Build history of the part. All positions in model axes, mm. Give positions to 0.01 mm unless a question says otherwise; leave off trailing zeros. Order: outer loops, then holes, each group sorted by start corner. A loop starts at its lowest first (then second) coordinate and runs counter-clockwise, first axis right, second up. Notation, with made-up numbers: (65, 0.25) - (88, 0.25) arc R36 cw to (88, 34.25) - close; hole circle Ø8 at (18.5, 70). An arc over 180 degrees is marked (long way). Write each question's results on one line, items separated by ' | '. Start each with the question number.
1) Cut at B-B on z = -7. List the corners of the cut face in (x, y).
2) Cut at C-C on y = 0. State how many separate pieces and enclosed holes the cut face has, plus the area to 3 significant figures.
3) Drill centre lines: line 1 along Z through (x, y) = (54, 10.75); line 2 along Z through (x, y) = (25.4, 11.6). Where is each one in solid material? Low to high. Write a range as from..to.
4) Two-plate mould, pull along Z, no slides. Class faces 1 (the face through (2, -12.7, -3)), 2 (the face through (-48.5, 11.9, 0.95)): +Z half, -Z half, draft (parallel to the pull), parting line (faces both ways), or undercut.
5) Drop a flat-ended pin along its axis: pin 1 Ø5.5 at (x, y) = (101.6, 0) entering from -Z. Give the stop position or say it passes through.
6) Cut at A-A on x = -101.6. List the corners of the cut face in (y, z).
from build123d import *

# Parameters (mm, degrees)
SKETCH1_W             = 25.4
SKETCH1_H             = 25.4
SKETCH1_W_2           = 22.225
SKETCH1_H_2           = 22.225
BOSS_EXTRUDE1_DEPTH   = 139.7
SKETCH3_W             = 2.4892
SKETCH3_H             = 25.4
SKETCH3_AT_POINT_2_W  = 2.4892
SKETCH3_AT_POINT_2_H  = 25.4
LPATTERN1_START       = -12.7
LPATTERN1_OUTLINE_R   = 2.4892
LPATTERN1_DEPTH       = 25.4
LPATTERN1_2_OUTLINE_R = 2.4892
LPATTERN1_2_DEPTH     = 25.4


# Read off the part's stored shape, not the designer's step: LPattern1
with BuildPart() as part:
    # Sketch1 → Boss-Extrude1 (new, symmetric)
    with BuildSketch(Plane(origin=(0, 0, 0), x_dir=(0, 0, -1), z_dir=(1, 0, 0))):
        Rectangle(SKETCH1_W, SKETCH1_H)
        Rectangle(SKETCH1_W_2, SKETCH1_H_2, mode=Mode.SUBTRACT)
    extrude(amount=BOSS_EXTRUDE1_DEPTH, both=True)

    # Sketch3 → #9 (0.196) Diameter Hole1 (revolve, cut)
    with BuildSketch(Plane(origin=(127, 12.7, 0), x_dir=(0, 0, 1), z_dir=(1, 0, 0))):
        with Locations((1.2446, 12.7)):
            Rectangle(SKETCH3_W, SKETCH3_H)
    revolve(axis=Axis((127, 19.05, 0), (0, -1, 0)), mode=Mode.SUBTRACT)

    # Sketch3 at point 2 (carried to point 2, square into its face) → #9 (0.196) Diameter Hole1 at 2 (revolve, cut)
    with BuildSketch(Plane(origin=(127, 0, 12.7), x_dir=(0, -1, 0), z_dir=(1, 0, 0))):
        with Locations((1.2446, 12.7)):
            Rectangle(SKETCH3_AT_POINT_2_W, SKETCH3_AT_POINT_2_H)
    revolve(axis=Axis((127, 0, 19.05), (0, 0, -1)), mode=Mode.SUBTRACT)

    # LPattern1 outline → LPattern1 (cut)
    with BuildSketch(Plane.XY.offset(LPATTERN1_START)):
        with Locations((101.6, 0)):
            Circle(LPATTERN1_OUTLINE_R)
        with Locations((76.2, 0)):
            Circle(LPATTERN1_OUTLINE_R)
        with Locations((50.8, 0)):
            Circle(LPATTERN1_OUTLINE_R)
        with Locations((25.4, 0)):
            Circle(LPATTERN1_OUTLINE_R)
        Circle(LPATTERN1_OUTLINE_R)
        with Locations((-25.4, 0)):
            Circle(LPATTERN1_OUTLINE_R)
        with Locations((-50.8, 0)):
            Circle(LPATTERN1_OUTLINE_R)
        with Locations((-76.2, 0)):
            Circle(LPATTERN1_OUTLINE_R)
        with Locations((-101.6, 0)):
            Circle(LPATTERN1_OUTLINE_R)
        with Locations((-127, 0)):
            Circle(LPATTERN1_OUTLINE_R)
    extrude(amount=LPATTERN1_DEPTH, mode=Mode.SUBTRACT)

    # LPattern1 2 outline → LPattern1 2 (cut)
    with BuildSketch(Plane(origin=(0, 0, 0), x_dir=(1, 0, 0), z_dir=(0, 1, 0)).offset(LPATTERN1_START)):
        with Locations((101.6, 0)):
            Circle(LPATTERN1_2_OUTLINE_R)
        with Locations((76.2, 0)):
            Circle(LPATTERN1_2_OUTLINE_R)
        with Locations((50.8, 0)):
            Circle(LPATTERN1_2_OUTLINE_R)
        with Locations((25.4, 0)):
            Circle(LPATTERN1_2_OUTLINE_R)
        Circle(LPATTERN1_2_OUTLINE_R)
        with Locations((-25.4, 0)):
            Circle(LPATTERN1_2_OUTLINE_R)
        with Locations((-50.8, 0)):
            Circle(LPATTERN1_2_OUTLINE_R)
        with Locations((-76.2, 0)):
            Circle(LPATTERN1_2_OUTLINE_R)
        with Locations((-101.6, 0)):
            Circle(LPATTERN1_2_OUTLINE_R)
        with Locations((-127, 0)):
            Circle(LPATTERN1_2_OUTLINE_R)
    extrude(amount=LPATTERN1_2_DEPTH, mode=Mode.SUBTRACT)


solid = part.part
Results:
1) outline: (-139.7, -12.7) - (139.7, -12.7) - (139.7, -11.11) - (-139.7, -11.11) - close; (-139.7, 11.11) - (139.7, 11.11) - (139.7, 12.7) - (-139.7, 12.7) - close
2) separate pieces: 24 | enclosed holes: 0 | area: 713 mm^2
3) line 1: -12.7..-11.11, 11.11..12.7 | line 2: -12.7..-2.49, 2.49..12.7
4) face 1: draft | face 2: undercut
5) pin 1: z = -12.7
6) outline: (-12.7, -12.7) - (-2.49, -12.7) - (-2.49, -11.11) - (-11.11, -11.11) - (-11.11, -2.49) - (-12.7, -2.49) - close; (-12.7, 2.49) - (-11.11, 2.49) - (-11.11, 11.11) - (-2.49, 11.11) - (-2.49, 12.7) - (-12.7, 12.7) - close; (2.49, -12.7) - (12.7, -12.7) - (12.7, -2.49) - (11.11, -2.49) - (11.11, -11.11) - (2.49, -11.11) - close; (2.49, 11.11) - (11.11, 11.11) - (11.11, 2.49) - (12.7, 2.49) - (12.7, 12.7) - (2.49, 12.7) - close
